```python
from build123d import *

# Parameters (mm, degrees)
F0_R      = 71.5350962672
F1_DEPTH  = 25.4
F4_W      = 16.7800951749
F4_H      = 74.4879245758
F4_W_2    = 16.4273940027
F5_DEPTH  = 25.4
F6_W      = 176.0196238756
F6_H      = 16.4934694767
F7_DEPTH  = 25.4
F8_W      = 33.9048393071
F8_H      = 156.475931406
F9_DEPTH  = 25.4
F11_DEPTH = 25.4


# Not quite as in the source:
# - the program builds the solid bodies; features that only make, move or delete a surface that nothing else refers to are left out


with BuildPart() as f1:
    # F0 (on Front) → F1 (new body)
    with BuildSketch(Plane.XZ):
        Circle(F0_R)
    extrude(amount=F1_DEPTH)

    # F4 (on Front) → F5 (join)
    with BuildSketch(Plane.XZ):
        with Locations((-8.3900475875, -108.3736568689)):
            Rectangle(F4_W, F4_H)
        with Locations((8.2136970013, -108.3736568689)):
            Rectangle(F4_W_2, F4_H)
    extrude(amount=F5_DEPTH)

    # F6 (on Front) → F7 (join)
    with BuildSketch(Plane.XZ):
        with Locations((0, -151.0558873415)):
            Rectangle(F6_W, F6_H)
    extrude(amount=F7_DEPTH)

    # F8 (on Front) → F9 (join)
    with BuildSketch(Plane.XZ):
        with Locations((0, -158.9946001768)):
            Rectangle(F8_W, F8_H)
    extrude(amount=F9_DEPTH)

    # F10 (on Front) → F11 (join)
    with BuildSketch(Plane.XZ):
        Polygon((46.7250607908, -236.9969040155), (0, -236.9969040155), (-43.9401827753, -236.9969040155), (-43.9401827753, -266.2233710289), (-44.8115989566, -287.0510220528), (-25.0311624259, -287.0510220528), (-25.0311624259, -259.9867582321), (30.4474048316, -259.9867582321), (30.4474048316, -289.1219854355), (46.7250607908, -289.1219854355), align=None)
    extrude(amount=F11_DEPTH)


solid = f1.part
```
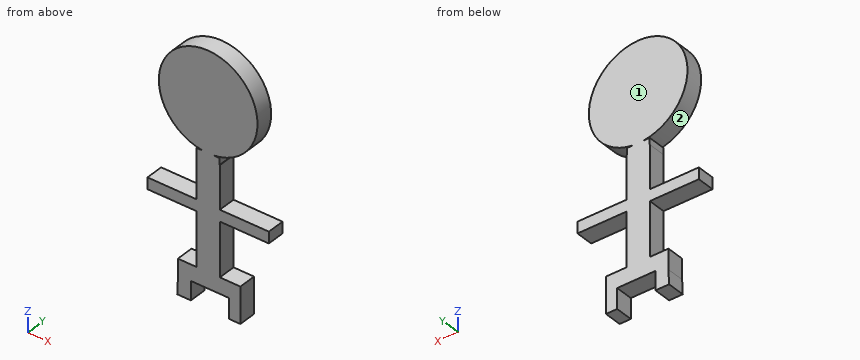
Can you work these out from the model? Positions are in its coordinate system, mm. Face numbers are marked on the shaded views. Give positions to 0.01 mm unless a question says otherwise; leave off trailing zeros. Write each loop counter-clockwise with the first axis right and the second up, starting at its lowest first coordinate (ties: lowest second). Pieces come first, ordered by that corner, then holes. Notation, with made-up numbers: (70, 85.5) -> (105, 85.5) arc R26 cw to (105, 123.5) -> close; hole circle Ø6 at (89, 74). An arc over 180 degrees is marked (long way). Write item = value, one per line.
(1) Suppose I cut it at A-A on x = 42. Write out the boundary of the cut face in (y, z).
Worked out:
outline = (-25.4, -289.12) -> (0, -289.12) -> (0, -237) -> (-25.4, -237) -> close; (-25.4, -159.3) -> (0, -159.3) -> (0, -142.81) -> (-25.4, -142.81) -> close; (-25.4, -57.91) -> (0, -57.91) -> (0, 57.91) -> (-25.4, 57.91) -> close
(2) I need wall thicknesses on probe 1 along Z at (x, y) = (21.5, -19.75); probe 2 along Z at (x, y) = (-23, -21.5); probe 3 along X at (y, z) = (-11.75, -261). Which ranges of each line are inside material? Lowest first, please. Write a range as from..to.
Worked out:
probe_1 = -259.99..-237, -159.3..-142.81, -68.23..68.23
probe_2 = -259.99..-237, -159.3..-142.81, -67.74..67.74
probe_3 = -43.94..-25.03, 30.45..46.73
(3) I'm going to push flat-ended pins straight in: P1, Ø10, axis at y = -21.5, z = 25, coming from the +X side; P2, Ø12.5, axis at y = -18.5, z = -181.5, coming from the +X side; P3, Ø3, axis at y = -16.5, z = -74, coming from the -X side; P4, Ø3, axis at y = -17.5, z = -159.5, coming from the -X side. Where does each tip first touch, or does it pass through?
Worked out:
P1 = 68.68
P2 = 16.95
P3 = -16.78
P4 = -88.01
(4) Suppose I cut it at B-B on y = -6. Write out the boundary of the cut face in (x, z).
Worked out:
outline = (-88.01, -159.3) -> (-16.95, -159.3) -> (-16.95, -237) -> (-43.94, -237) -> (-43.94, -266.22) -> (-44.81, -287.05) -> (-25.03, -287.05) -> (-25.03, -259.99) -> (30.45, -259.99) -> (30.45, -289.12) -> (46.73, -289.12) -> (46.73, -237) -> (16.95, -237) -> (16.95, -159.3) -> (88.01, -159.3) -> (88.01, -142.81) -> (16.95, -142.81) -> (16.95, -80.76) -> (16.43, -80.76) -> (16.43, -71.13) -> (7.61, -71.13) arc R71.54 ccw (long way) to (-7.61, -71.13) -> (-16.78, -71.13) -> (-16.78, -80.76) -> (-16.95, -80.76) -> (-16.95, -142.81) -> (-88.01, -142.81) -> close
(5) Suppose I cut it at C-C on z = 0. Write out the boundary of the cut face in (x, y).
Worked out:
outline = (-71.54, -25.4) -> (71.54, -25.4) -> (71.54, 0) -> (-71.54, 0) -> close
(6) Suppose I cut it at D-D on x = 0. Write out the boundary of the cut face in (y, z).
Worked out:
outline = (-25.4, -259.99) -> (0, -259.99) -> (0, 71.54) -> (-25.4, 71.54) -> close
(7) Thinking about a two-plate mould opening in Z: for the marked faces 1 and 2, which applies, released by +Z, released by -Z, zero draft, split by the parting line, or undercut?
Worked out:
face_1 = zero draft
face_2 = undercut
